```python
from build123d import *

# Parameters (mm, degrees)
BOSS_EXTRUDE1_DEPTH = 3
CUT_EXTRUDE1_REACH  = 66.915
SKETCH2_R           = 4.25
SKETCH2_R_2         = 1.05
SKETCH3_R           = 1.9
CUT_EXTRUDE2_DEPTH  = 1
BOSS_EXTRUDE2_DEPTH = 29
BOSS_EXTRUDE4_DEPTH = 3
CUT_EXTRUDE3_REACH  = 165.217
SKETCH8_R           = 1.05
SKETCH9_R           = 1.9
CUT_EXTRUDE4_DEPTH  = 1
CUT_EXTRUDE5_REACH  = 165.539
BOSS_EXTRUDE8_REACH = 166.778
SKETCH16_W          = 3.2
SKETCH16_H          = 2
CUT_EXTRUDE6_DEPTH  = 166.80352831
CUT_EXTRUDE7_REACH  = 166.778
SKETCH17_W          = 7
SKETCH17_H          = 11
SKETCH18_W          = 25
SKETCH18_H          = 3
CUT_EXTRUDE8_DEPTH  = 21


with BuildPart() as part:
    # Sketch1 → Boss-Extrude1 (new body)
    with BuildSketch(Plane.XY):
        with BuildLine():
            Line((25, 29), (48.666332079, 25.373055569))
            ThreePointArc((48.666332079, 25.373055569), (58, 14.5), (48.666332079, 3.626944431))
            Line((48.666332079, 3.626944431), (25, 0))
            Line((25, 0), (0, 0))
            Line((0, 0), (0, 29))
            Line((0, 29), (25, 29))
        make_face()
    extrude(amount=-BOSS_EXTRUDE1_DEPTH)

    # Sketch2 → Cut-Extrude1 (cut, up to next)
    with BuildSketch(Plane.XY, mode=Mode.PRIVATE) as cut_extrude1_sk1:
        with Locations((47, 14.5)):
            Circle(SKETCH2_R)
    cut_extrude1_tool1 = extrude(cut_extrude1_sk1.sketch, amount=-CUT_EXTRUDE1_REACH, mode=Mode.PRIVATE) & part.part
    # Sketch2 → Cut-Extrude1 (cut, up to next)
    with BuildSketch(Plane.XY, mode=Mode.PRIVATE) as cut_extrude1_sk2:
        with Locations((47, 22.5)):
            Circle(SKETCH2_R_2)
    cut_extrude1_tool2 = extrude(cut_extrude1_sk2.sketch, amount=-CUT_EXTRUDE1_REACH, mode=Mode.PRIVATE) & part.part
    # Sketch2 → Cut-Extrude1 (cut, up to next)
    with BuildSketch(Plane.XY, mode=Mode.PRIVATE) as cut_extrude1_sk3:
        with Locations((55, 14.5)):
            Circle(SKETCH2_R_2)
    cut_extrude1_tool3 = extrude(cut_extrude1_sk3.sketch, amount=-CUT_EXTRUDE1_REACH, mode=Mode.PRIVATE) & part.part
    # Sketch2 → Cut-Extrude1 (cut, up to next)
    with BuildSketch(Plane.XY, mode=Mode.PRIVATE) as cut_extrude1_sk4:
        with Locations((47, 6.5)):
            Circle(SKETCH2_R_2)
    cut_extrude1_tool4 = extrude(cut_extrude1_sk4.sketch, amount=-CUT_EXTRUDE1_REACH, mode=Mode.PRIVATE) & part.part
    # Sketch2 → Cut-Extrude1 (cut, up to next)
    with BuildSketch(Plane.XY, mode=Mode.PRIVATE) as cut_extrude1_sk5:
        with Locations((39, 14.5)):
            Circle(SKETCH2_R_2)
    cut_extrude1_tool5 = extrude(cut_extrude1_sk5.sketch, amount=-CUT_EXTRUDE1_REACH, mode=Mode.PRIVATE) & part.part
    add(cut_extrude1_tool1.solids().sort_by_distance((47, 14.5, 0))[0], mode=Mode.SUBTRACT)
    add(cut_extrude1_tool2.solids().sort_by_distance((47, 22.5, 0))[0], mode=Mode.SUBTRACT)
    add(cut_extrude1_tool3.solids().sort_by_distance((55, 14.5, 0))[0], mode=Mode.SUBTRACT)
    add(cut_extrude1_tool4.solids().sort_by_distance((47, 6.5, 0))[0], mode=Mode.SUBTRACT)
    add(cut_extrude1_tool5.solids().sort_by_distance((39, 14.5, 0))[0], mode=Mode.SUBTRACT)

    # Sketch3 → Cut-Extrude2 (cut)
    with BuildSketch(Plane.XY):
        with Locations((47, 22.5)):
            Circle(SKETCH3_R)
        with Locations((55, 14.5)):
            Circle(SKETCH3_R)
        with Locations((47, 6.5)):
            Circle(SKETCH3_R)
        with Locations((39, 14.5)):
            Circle(SKETCH3_R)
    extrude(amount=-CUT_EXTRUDE2_DEPTH, mode=Mode.SUBTRACT)

    # Sketch4 → Boss-Extrude2 (add)
    with BuildSketch(Plane(origin=(0, 29, 0), x_dir=(1, 0, 0), z_dir=(0, 1, 0))):
        Polygon((0, 3), (0, 0), (-30, 10), (-110, 10), (-140, 5), (-140, 8), (-110, 13), (-30, 13), align=None)
    extrude(amount=-BOSS_EXTRUDE2_DEPTH)

    # Sketch7 → Boss-Extrude4 (add)
    with BuildSketch(Plane.XY.offset(-5)):
        Polygon((-140, 29), (-144.7, 33.7), (-159.5, 33.7), (-159.5, 25), (-146, 25), (-146, 4), (-159.5, 4), (-159.5, -4.7), (-144.7, -4.7), (-140, 0), align=None)
    extrude(amount=-BOSS_EXTRUDE4_DEPTH)

    # Sketch8 → Cut-Extrude3 (cut, up to next)
    with BuildSketch(Plane.XY.offset(-5), mode=Mode.PRIVATE) as cut_extrude3_sk1:
        with Locations((-156.25, 28)):
            Circle(SKETCH8_R)
    cut_extrude3_tool1 = extrude(cut_extrude3_sk1.sketch, amount=-CUT_EXTRUDE3_REACH, mode=Mode.PRIVATE) & part.part
    # Sketch8 → Cut-Extrude3 (cut, up to next)
    with BuildSketch(Plane.XY.offset(-5), mode=Mode.PRIVATE) as cut_extrude3_sk2:
        with Locations((-148.25, 28)):
            Circle(SKETCH8_R)
    cut_extrude3_tool2 = extrude(cut_extrude3_sk2.sketch, amount=-CUT_EXTRUDE3_REACH, mode=Mode.PRIVATE) & part.part
    # Sketch8 → Cut-Extrude3 (cut, up to next)
    with BuildSketch(Plane.XY.offset(-5), mode=Mode.PRIVATE) as cut_extrude3_sk3:
        with Locations((-143, 22.5)):
            Circle(SKETCH8_R)
    cut_extrude3_tool3 = extrude(cut_extrude3_sk3.sketch, amount=-CUT_EXTRUDE3_REACH, mode=Mode.PRIVATE) & part.part
    # Sketch8 → Cut-Extrude3 (cut, up to next)
    with BuildSketch(Plane.XY.offset(-5), mode=Mode.PRIVATE) as cut_extrude3_sk4:
        with Locations((-143, 6.5)):
            Circle(SKETCH8_R)
    cut_extrude3_tool4 = extrude(cut_extrude3_sk4.sketch, amount=-CUT_EXTRUDE3_REACH, mode=Mode.PRIVATE) & part.part
    # Sketch8 → Cut-Extrude3 (cut, up to next)
    with BuildSketch(Plane.XY.offset(-5), mode=Mode.PRIVATE) as cut_extrude3_sk5:
        with Locations((-148.25, 1)):
            Circle(SKETCH8_R)
    cut_extrude3_tool5 = extrude(cut_extrude3_sk5.sketch, amount=-CUT_EXTRUDE3_REACH, mode=Mode.PRIVATE) & part.part
    # Sketch8 → Cut-Extrude3 (cut, up to next)
    with BuildSketch(Plane.XY.offset(-5), mode=Mode.PRIVATE) as cut_extrude3_sk6:
        with Locations((-156.25, 1)):
            Circle(SKETCH8_R)
    cut_extrude3_tool6 = extrude(cut_extrude3_sk6.sketch, amount=-CUT_EXTRUDE3_REACH, mode=Mode.PRIVATE) & part.part
    add(cut_extrude3_tool1.solids().sort_by_distance((-156.25, 28, -5))[0], mode=Mode.SUBTRACT)
    add(cut_extrude3_tool2.solids().sort_by_distance((-148.25, 28, -5))[0], mode=Mode.SUBTRACT)
    add(cut_extrude3_tool3.solids().sort_by_distance((-143, 22.5, -5))[0], mode=Mode.SUBTRACT)
    add(cut_extrude3_tool4.solids().sort_by_distance((-143, 6.5, -5))[0], mode=Mode.SUBTRACT)
    add(cut_extrude3_tool5.solids().sort_by_distance((-148.25, 1, -5))[0], mode=Mode.SUBTRACT)
    add(cut_extrude3_tool6.solids().sort_by_distance((-156.25, 1, -5))[0], mode=Mode.SUBTRACT)

    # Sketch9 → Cut-Extrude4 (cut)
    with BuildSketch(Plane.XY.offset(-5)):
        with Locations((-156.25, 28)):
            Circle(SKETCH9_R)
        with Locations((-148.25, 28)):
            Circle(SKETCH9_R)
        with Locations((-143, 22.5)):
            Circle(SKETCH9_R)
        with Locations((-143, 6.5)):
            Circle(SKETCH9_R)
        with Locations((-148.25, 1)):
            Circle(SKETCH9_R)
        with Locations((-156.25, 1)):
            Circle(SKETCH9_R)
    extrude(amount=-CUT_EXTRUDE4_DEPTH, mode=Mode.SUBTRACT)

    # Cut-Extrude5: up to this face of the body (flat: up to its plane)
    cut_extrude5_end = Plane(part.part.faces().sort_by_distance((-70, 14.5, -13))[0])
    # Sketch11 → Cut-Extrude5 (cut, up to the picked face)
    with BuildSketch(Plane.XY, mode=Mode.PRIVATE) as cut_extrude5_sk1:
        Polygon((0, 0), (-30, 2), (-110, 2), (-140, 0), align=None)
    cut_extrude5_tool1 = split(extrude(cut_extrude5_sk1.sketch, amount=-CUT_EXTRUDE5_REACH, mode=Mode.PRIVATE), bisect_by=cut_extrude5_end, keep=Keep.BOTH, mode=Mode.PRIVATE)
    # Sketch11 → Cut-Extrude5 (cut, up to the picked face)
    with BuildSketch(Plane.XY, mode=Mode.PRIVATE) as cut_extrude5_sk2:
        Polygon((0, 29), (-30, 27), (-110, 27), (-140, 29), align=None)
    cut_extrude5_tool2 = split(extrude(cut_extrude5_sk2.sketch, amount=-CUT_EXTRUDE5_REACH, mode=Mode.PRIVATE), bisect_by=cut_extrude5_end, keep=Keep.BOTH, mode=Mode.PRIVATE)
    add(cut_extrude5_tool1.solids().sort_by(Axis((-70, 0.909091, 0), (0, 0, -1)))[0], mode=Mode.SUBTRACT)
    add(cut_extrude5_tool2.solids().sort_by(Axis((-70, 28.090909, 0), (0, 0, -1)))[0], mode=Mode.SUBTRACT)

    # Sketch14 → Boss-Extrude8 (add, up to next)
    with BuildSketch(Plane.XY.offset(-24), mode=Mode.PRIVATE) as boss_extrude8_sk1:
        Polygon((-159.5, 33.7), (-159.5, 30.7), (-144.7, 30.7), (-140, 26), (-110, 24), (-30, 24), (0, 26), (25, 26), (25, 29), (0, 29), (-30, 27), (-110, 27), (-140, 29), (-144.7, 33.7), align=None)
    boss_extrude8_tool1 = extrude(boss_extrude8_sk1.sketch, amount=BOSS_EXTRUDE8_REACH, mode=Mode.PRIVATE) - part.part
    boss_extrude8 = boss_extrude8_tool1.solids().sort_by_distance((-67.25, 26.744472, -24))[0]
    add(boss_extrude8)

    # Mirror1: Boss-Extrude8 across plane
    add(boss_extrude8.mirror(Plane.ZX.offset(14.5)))

    # Sketch16 → Cut-Extrude6 (cut, through all)
    with BuildSketch(Plane(origin=(0, 33.7, 0), x_dir=(1, 0, 0), z_dir=(0, 1, 0))):
        with Locations((-152.9, 20)):
            Rectangle(SKETCH16_W, SKETCH16_H)
        with Locations((-70, 20)):
            Rectangle(SKETCH16_W, SKETCH16_H)
        with Locations((10.6, 20)):
            Rectangle(SKETCH16_W, SKETCH16_H)
    extrude(amount=-CUT_EXTRUDE6_DEPTH, mode=Mode.SUBTRACT)

    # Sketch17 → Cut-Extrude7 (cut, up to next)
    with BuildSketch(Plane.XY, mode=Mode.PRIVATE) as cut_extrude7_sk1:
        with Locations((-131.5, 14.5)):
            Rectangle(SKETCH17_W, SKETCH17_H)
    cut_extrude7_tool1 = extrude(cut_extrude7_sk1.sketch, amount=-CUT_EXTRUDE7_REACH, mode=Mode.PRIVATE) & part.part
    # Sketch17 → Cut-Extrude7 (cut, up to next)
    with BuildSketch(Plane.XY, mode=Mode.PRIVATE) as cut_extrude7_sk2:
        with Locations((16.5, 14.5)):
            Rectangle(SKETCH17_W, SKETCH17_H)
    cut_extrude7_tool2 = extrude(cut_extrude7_sk2.sketch, amount=-CUT_EXTRUDE7_REACH, mode=Mode.PRIVATE) & part.part
    add(cut_extrude7_tool1.solids().sort_by_distance((-131.5, 14.5, 0))[0], mode=Mode.SUBTRACT)
    add(cut_extrude7_tool2.solids().sort_by_distance((16.5, 14.5, 0))[0], mode=Mode.SUBTRACT)

    # Sketch18 → Cut-Extrude8 (cut)
    with BuildSketch(Plane(origin=(0, 0, -24), x_dir=(-1, 0, 0), z_dir=(0, 0, -1))):
        with Locations((-12.5, 27.5)):
            Rectangle(SKETCH18_W, SKETCH18_H)
    extrude(amount=-CUT_EXTRUDE8_DEPTH, mode=Mode.SUBTRACT)


solid = part.part
```
Here's how the part is built. I have some questions about the finished solid (model axes, mm). A direction names the side the tool comes from. Give positions to 0.01 mm unless a question says otherwise; leave off trailing zeros. Loops run counter-clockwise (first coordinate to the right, second up) from the corner with the lowest first, then second, coordinate; pieces in that order, holes last. Notation, with made-up numbers: M -8.75,68.5 L 18.25,68.5 A21 ccw 18.25,104.5 Z; hole C -28.75,49 d7. An arc over 180 degrees is marked long. Put each result on its own line as item: value. Start each with the question number.
(1) I want a section at A-A on z = -16.5. Please give me the cut outline in (x, y).
(2) If we mould it in two halves opening along X, with no side actions, what happens to faces 4 (the flat face through (-124.79, 14.703, -7.535)), 5 (the flat face through (48.2, 22.5, -1)), 6 (the flat face through (-145.6, 14.8, -5)), 7 (the flat face through (-142, 31, -15))? For each: +X half, -X half, draft (parallel to the pull), parting line (faces both ways), or undercut.
(3) I want a section at C-C on x = -41.5. Please give me the cut outline in (y, z), then the cut area to 3 significant figures.
(4) I want a section at B-B on x = -10.5. Please give me the cut outline in (y, z).
(5) I need wall thicknesses on line 1 along Y through (x, z) = (-148.25, -5.5); line 2 along Y through (x, z) = (-148.25, -7.15); line 3 along Y through (x, z) = (-55, -19.25). Which ranges of each line are inside material? Lowest first, please. Write a range as [from, to].
(6) Will these pins go through, and if not, where does the flat tip stop? pin 1 Ø1.5 at (y, z) = (13.5, -14.5) entering from +X; pin 2 Ø1.5 at (y, z) = (29.5, -11.5) entering from -X; pin 3 Ø3.5 at (x, y) = (-148.25, 1) entering from +Z; pin 4 Ø6.5 at (x, z) = (18.5, -10.5) entering from +Y.
(7) For faces 1 (the cylindrical face through (48.812, 23.071, -0.493)), 2 (the flat face through (-69, 27, -17)), 3 (the flat face through (-69, 15, -10)), which set-ups out of +Z, -Z, +X, -X, +Y, -Y let a thin tool reach every point of the face, with its end or its side?
Answer block:
1. outline: M -159.5,-4.7 L -144.7,-4.7 L -140,0 L -110,2 L -30,2 L 0,0 L 25,0 L 25,3 L 0,3 L -30,5 L -110,5 L -140,3 L -144.7,-1.7 L -159.5,-1.7 Z; M -159.5,30.7 L -144.7,30.7 L -140,26 L -110,24 L -30,24 L 0,26 L 0,29 L -30,27 L -110,27 L -140,29 L -144.7,33.7 L -159.5,33.7 Z
2. face 4: undercut
2. face 5: undercut
2. face 6: draft
2. face 7: +X half
3. outline: M 2,-24 L 5,-24 L 5,-13 L 24,-13 L 24,-24 L 27,-24 L 27,-10 L 2,-10 Z
3. area: 141 mm^2
4. outline: M 0.7,-24 L 3.7,-24 L 3.7,-6.5 L 25.3,-6.5 L 25.3,-24 L 28.3,-24 L 28.3,-3.5 L 0.7,-3.5 Z
5. line 1: [-4.7, -0.9], [2.9, 4], [25, 26.1], [29.9, 33.7]
5. line 2: [-4.7, -0.05], [2.05, 4], [25, 26.95], [29.05, 33.7]
5. line 3: [2, 5], [24, 27]
6. pin 1: through
6. pin 2: x = -144.25
6. pin 3: z = -6
6. pin 4: y = 3
7. face 1: +Z
7. face 2: +Z, -Z, +Y
7. face 3: +Z, +Y, -Y
